Source: CAD feature listing. Evaluate the final solid. Frame: model axes, mm. Give positions to 0.01 mm unless a question says otherwise; leave off trailing zeros. Order: outer loops, then holes, each group sorted by start corner. A loop starts at its lowest first (then second) coordinate and runs counter-clockwise, first axis right, second up. Notation, with made-up numbers: (37, -27.5) - (95, -27.5) arc R21 cw to (95, -21.5) - close; hole circle Ø7 at (-0.5, 50.5). An arc over 180 degrees is marked (long way). Use CSV: the item, a comma, the result in double quotes.
Solid Edge part; units mm, degrees
sketch "Sketch1" plane through (0, 0, 0) normal (0, 0, 1) x (1, 0, 0)
  line L0 (-105, -61.5) -> (105, -61.5)
  line L1 (105, -61.5) -> (105, 61.5)
  line L2 (105, 61.5) -> (-105, 61.5)
  line L3 (-105, 61.5) -> (-105, -61.5)
  dimension "D1" = 105
  dimension "D2" = 105
extrude "Protrusion1" add sketch "Sketch1" along normal blind 2
hole "Hole1" at (73, -52.5, 2) direction (0, 0, -1) diameter 1 end through all
hole "Hole2" at (73, -30.5, 2) direction (0, 0, -1) diameter 1 end through all
hole "Hole3" at (73, -8.5, 2) direction (0, 0, -1) diameter 1 end through all
hole "Hole4" at (95, -8.5, 2) direction (0, 0, -1) diameter 1 end through all
hole "Hole5" at (95, -30.5, 2) direction (0, 0, -1) diameter 1 end through all
hole "Hole6" at (73, 13.5, 2) direction (0, 0, -1) diameter 1 end through all
hole "Hole7" at (95, -52.5, 2) direction (0, 0, -1) diameter 1 end through all
sketch "Sketch2" plane through (0, 0, 2) normal (0, 0, 1) x (1, 0, 0)
  line L0 (65.5, 22.5) -> (80.5, 22.5)
  line L1 (80.5, 22.5) -> (80.5, 24.5)
  line L2 (80.5, 24.5) -> (65.5, 24.5)
  line L3 (65.5, 24.5) -> (65.5, 22.5)
  dimension "D1" = 80.5
  dimension "D2" = 65.5
extrude "Cutout1" cut sketch "Sketch2" against normal through all
sketch "Sketch3" plane through (0, 0, 2) normal (0, 0, 1) x (1, 0, 0)
  line L0 (-105, -61.5) -> (50, -61.5)
  line L1 (50, 2.5) -> (50, -61.5)
  line L2 (59, 2.5) -> (50, 2.5)
  line L3 (59, 24.5) -> (59, 2.5)
  line L4 (50, 24.5) -> (59, 24.5)
  line L5 (50, 61.5) -> (50, 24.5)
  line L6 (50, 61.5) -> (-105, 61.5)
  line L7 (-105, 61.5) -> (-105, -61.5)
  dimension "D1" = 50
  dimension "D2" = 59
extrude "Ausschnitt_3" cut sketch "Sketch3" against normal blind 2
hole "Hole8" at (98.5, 49.5, 2) direction (0, 0, -1) diameter 3.5 end through all
hole "Hole9" at (98.5, -41.5, 2) direction (0, 0, -1) diameter 3.5 end through all
hole "Hole10" at (55, -56.5, 2) direction (0, 0, -1) diameter 3.5 end through all
hole "Hole11" at (98.5, 5.5, 2) direction (0, 0, -1) diameter 3.5 end through all
hole "Hole12" at (55, 28.5, 2) direction (0, 0, -1) diameter 3.5 end through all
hole "Befestigungsbohrung_Plus" at (103, -41.5, 2) direction (0, 0, -1) diameter 3.5 end through all
hole "Hole13" at (54, -42.5, 2) direction (0, 0, -1) diameter 1 end through all
hole "Inkrementalgeber" at (95, 25.5, 2) direction (0, 0, -1) diameter 1 end through all
hole "Hole14" at (81.5, -43.5, 2) direction (0, 0, -1) diameter 1 end through all
hole "Hole15" at (81.5, -21.5, 2) direction (0, 0, -1) diameter 1 end through all
hole "Hole16" at (81.5, 0.5, 2) direction (0, 0, -1) diameter 1 end through all
hole "Hole17" at (86.5, 0.5, 2) direction (0, 0, -1) diameter 1 end through all
hole "Hole18" at (86.5, -43.5, 2) direction (0, 0, -1) diameter 1 end through all
Item 1: Section D-D on z = 1.55. Count the separate pieces of the cut face and the enclosed holes in it, then the cut area to 3 significant figures.
Filled in:
separate pieces,"1"
enclosed holes,"21"
area,"6,470 mm2"
Item 2: First-contact query: pin 1 (1 mm diameter, centred on y = 23, z = 0.5, fed in from -X). Flat tip, straight axial feed; report the tip coordinate or a pass-through.
Filled in:
pin 1,"stops at x = 59"
Item 3: Section C-C on x = 98.5. Return the cut outline in (y, z), then the cut area to 3 significant figures.
Filled in:
outline,"(-61.5, 0) - (-43.25, 0) - (-43.25, 2) - (-61.5, 2) - close; (-39.75, 0) - (3.75, 0) - (3.75, 2) - (-39.75, 2) - close; (7.25, 0) - (47.75, 0) - (47.75, 2) - (7.25, 2) - close; (51.25, 0) - (61.5, 0) - (61.5, 2) - (51.25, 2) - close"
area,"225 mm2"
Item 4: Section A-A on y = 5.5. Return the cut outline in (x, z), then the cut area to 3 significant figures.
Filled in:
outline,"(59, 0) - (96.75, 0) - (96.75, 2) - (59, 2) - close; (100.25, 0) - (105, 0) - (105, 2) - (100.25, 2) - close"
area,"85.0 mm2"
Item 5: Material intervals for line 1 (Y direction, x = 73, z = 0.8); line 2 (X direction, y = -41.5, z = 0.6); line 3 (Y direction, x = 98.5, z = 1.1), sorted ascending. Write a range as from..to.
Filled in:
line 1,"y = -61.5..-53, -52..-31, -30..-9, -8..13, 14..22.5, 24.5..61.5"
line 2,"x = 50..96.75, 100.25..101.25, 104.75..105"
line 3,"y = -61.5..-43.25, -39.75..3.75, 7.25..47.75, 51.25..61.5"
Item 6: Mould query, pull axis Y, two halves, no side actions, for faces 1 (the flat face through (77, 1, 0)), 2 (the cylindrical face through (97.83, 47.883, 1.014)). Classes: released by +Y, released by -Y, zero draft, split by the parting line, or undercut.
Filled in:
face 1,"zero draft"
face 2,"undercut"
Item 7: Section B-B on x = 79. Return the cut outline in (y, z), then the cut area to 3 significant figures.
Filled in:
outline,"(-61.5, 0) - (22.5, 0) - (22.5, 2) - (-61.5, 2) - close; (24.5, 0) - (61.5, 0) - (61.5, 2) - (24.5, 2) - close"
area,"242 mm2"
